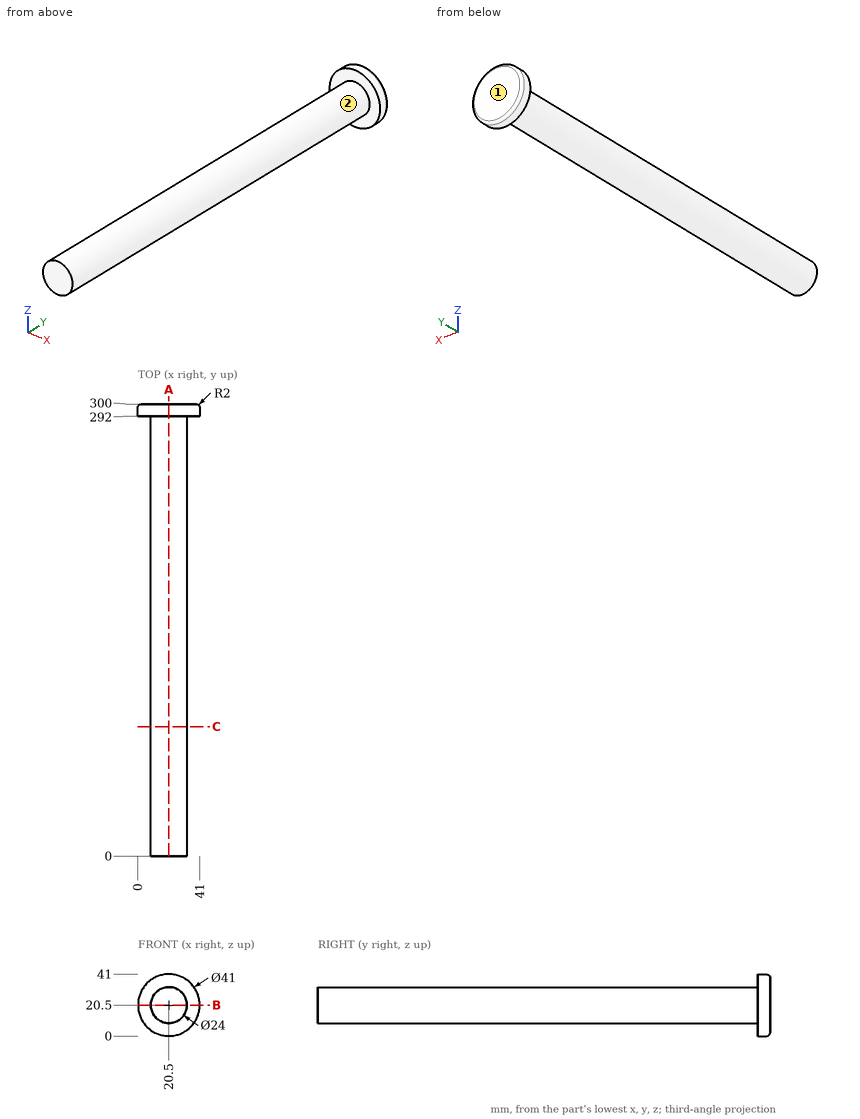
Design review of the part shown in the three views and the two pictorial views. Dimensions are in mm from the part's minimum x, y and z. A direction names the side the tool comes from. Round coordinates to 2 decimals unless told otherwise and drop trailing zeros. Loops run counter-clockwise (first coordinate to the right, second up) from the corner with the lowest first, then second, coordinate; pieces in that order, holes last. Notation, with made-up numbers: (-13.75, 64.25) -> (36.25, 64.25) arc R27 cw to (36.25, 102.25) -> close; hole circle Ø5 at (53, -33.75). An arc over 180 degrees is marked (long way). Answer as CSV lines item,"result".
1) Add section C-C on y = 86. Write out the cut boundary in (x, z).
Geometry results:
outline,"circle Ø24 at (20.5, 20.5)"
2) Add section B-B on z = 20.5. Write out the cut boundary in (x, y).
Geometry results:
outline,"(0, 292) -> (8.5, 292) -> (8.5, 0) -> (32.5, 0) -> (32.5, 292) -> (41, 292) -> (41, 298) arc R2 ccw to (39, 300) -> (2, 300) arc R2 ccw to (0, 298) -> close"
3) For P1, Ø5, axis at x = 22, y = 70.5, coming from the +Z side; P2, Ø1, axis at x = 12.5, y = 134.5, coming from the +Z side; P3, Ø10, axis at x = 7, y = 148, coming from the +Z side, all flat-tipped, find the tip position at first contact; note any pin that passes through.
Geometry results:
P1,"stops at z = 32.5"
P2,"stops at z = 29.87"
P3,"stops at z = 28.97"
4) To check wall thickness, follow line 1 along Y through (x, z) = (33, 7); line 2 along X through (y, z) = (134, 19); line 3 along Z through (x, y) = (15, 65). State the ranges of each line that lie inside material, in increasing order. Write a range as from..to.
Geometry results:
line 1,"y = 292..300"
line 2,"x = 8.59..32.41"
line 3,"z = 9.83..31.17"
5) Add section A-A on x = 20.5. Write out the cut boundary in (y, z).
Geometry results:
outline,"(0, 8.5) -> (292, 8.5) -> (292, 0) -> (298, 0) arc R2 ccw to (300, 2) -> (300, 39) arc R2 ccw to (298, 41) -> (292, 41) -> (292, 32.5) -> (0, 32.5) -> close"
6) Tool access review of the marked faces 1 and 2: name each direction out of +Z, -Z, +X, -X, +Y, -Y from which nothing blocks a thin tool from reaching the whole face with its end or side.
Geometry results:
face 1,"+Z, -Z, +X, -X, +Y"
face 2,"-Y"
